For this review, take the finished solid that the model builds, in its own axes (mm). A direction names the side the tool comes from. Coordinates: 2 decimals unless noted, no trailing zeros. Write each loop counter-clockwise with the first axis right and the second up, starting at its lowest first coordinate (ties: lowest second). Pieces come first, ordered by that corner, then holes. Notation, with made-up numbers: (-13, 27) -> (-5, 27) arc R33 cw to (-5, 58) -> close; hole circle Ø11 at (29.25, 75.25). An arc over 180 degrees is marked (long way). One line per item, written item: value. Start each with the question number.
1) Mouldability with a two-part tool opening along X and no side actions: class faces 3 (the flat face through (-46, 23, 0)), 4 (the flat face through (-1, 0, 0)), 5 (the cylindrical face through (82.23, 9.86, -23.46)) as released by +X, released by -X, zero draft, split by the parting line, or undercut.
2) For probe 1 along X at (y, z) = (15.75, 21.5); probe 2 along Z at (x, y) = (87.5, 11); probe 3 along Y at (x, z) = (77, 5.5), list the stretches that pass through material, from the lowest coordinate up. Write a range as from..to.
3) Add section A-A (z = -21.5). State the section outline as (x, y) points.
4) Add section B-B (x = 86). State the section outline as (y, z) points.
5) Add section D-D (z = 13). State the section outline as (x, y) points, and give its area (3 significant figures).
6) For pin 1 Ø11 at (x, z) = (43, 21.5) entering from +Y, flat-tipped, find the tip position at first contact; note if it passes through.
7) Machinability: for faces 1 (the flat face through (24, 20, 0)), 2 (the cylindrical face through (82.23, 9.86, 19.54)), which of the approach directions +Z, -Z, +X, -X, +Y, -Y give a long, thin tool a straight path to every point of the face, cutting with its end or side? Answer none if there is none.
8) Add section C-C (y = 2). State the section outline as (x, z) points, and give its area (3 significant figures).
from build123d import *

# Parameters (mm, degrees)
SKETCH_1_W                  = 192
SKETCH_1_H                  = 70
EXTRUDE_1_DEPTH             = 25
CUT_EXTRUDE_1_REACH         = 107.195
SKETCH_2_R                  = 4.25
PATTERN_LINEAR_1_COUNT      = 2
PATTERN_LINEAR_1_PITCH      = 43
PATTERN_LINEAR_1_COUNT_DIR2 = 2
PATTERN_LINEAR_1_PITCH_DIR2 = 43
SKETCH_3_W                  = 142
SKETCH_3_H                  = 70
CUT_EXTRUDE_2_DEPTH         = 5


with BuildPart() as part:
    # 草图1 → 凸台-拉伸1 (new body)
    with BuildSketch(Plane(origin=(0, 0, 0), x_dir=(1, 0, 0), z_dir=(0, 1, 0))):
        Rectangle(SKETCH_1_W, SKETCH_1_H)
    extrude(amount=EXTRUDE_1_DEPTH)

    # 草图2 → 切除-拉伸1 (cut, up to next)
    with BuildSketch(Plane.XZ, mode=Mode.PRIVATE) as cut_extrude_1_sk1:
        with Locations(Location((86, 21.5, 0), (0, 0, 270))):
            Circle(SKETCH_2_R)
    cut_extrude_1_tool1 = extrude(cut_extrude_1_sk1.sketch, amount=-CUT_EXTRUDE_1_REACH, mode=Mode.PRIVATE) & part.part
    cut_extrude_1 = cut_extrude_1_tool1.solids().sort_by_distance((86, 0, 21.5))[0]
    add(cut_extrude_1, mode=Mode.SUBTRACT)

    # 阵列(线性)1: Cut-Extrude 1 2 × 2
    with Locations(*[(-i * PATTERN_LINEAR_1_PITCH, 0, -j * PATTERN_LINEAR_1_PITCH_DIR2) for i in range(PATTERN_LINEAR_1_COUNT) for j in range(PATTERN_LINEAR_1_COUNT_DIR2) if (i, j) != (0, 0)]):
        add(cut_extrude_1, mode=Mode.SUBTRACT)

    # 草图3 → 切除-拉伸2 (cut)
    with BuildSketch(Plane(origin=(0, 25, 0), x_dir=(1, 0, 0), z_dir=(0, 1, 0))):
        with Locations((25, 0)):
            Rectangle(SKETCH_3_W, SKETCH_3_H)
    extrude(amount=-CUT_EXTRUDE_2_DEPTH, mode=Mode.SUBTRACT)


solid = part.part
Numbers:
1. face 3: released by +X
1. face 4: zero draft
1. face 5: undercut
2. probe 1: -96..38.75, 47.25..81.75, 90.25..96
2. probe 2: -35..-25.48, -17.52..17.52, 25.48..35
2. probe 3: 0..20
3. outline: (-96, 0) -> (38.75, 0) -> (38.75, 20) -> (-46, 20) -> (-46, 25) -> (-96, 25) -> close; (47.25, 0) -> (81.75, 0) -> (81.75, 20) -> (47.25, 20) -> close; (90.25, 0) -> (96, 0) -> (96, 20) -> (90.25, 20) -> close
4. outline: (0, -35) -> (20, -35) -> (20, -25.75) -> (0, -25.75) -> close; (0, -17.25) -> (20, -17.25) -> (20, 17.25) -> (0, 17.25) -> close; (0, 25.75) -> (20, 25.75) -> (20, 35) -> (0, 35) -> close
5. outline: (-96, 0) -> (96, 0) -> (96, 20) -> (-46, 20) -> (-46, 25) -> (-96, 25) -> close
5. area: 4,090 mm²
6. pin 1: y = 20
7. face 1: +Z, -Z, +X, +Y
7. face 2: +Y, -Y
8. outline: (-96, -35) -> (96, -35) -> (96, 35) -> (-96, 35) -> close; hole circle Ø8.5 at (43, -21.5); hole circle Ø8.5 at (43, 21.5); hole circle Ø8.5 at (86, -21.5); hole circle Ø8.5 at (86, 21.5)
8. area: 13,200 mm²
